from build123d import *

# Parameters (mm, degrees)
F0_W     = 370
F0_H     = 130
F1_DEPTH = 150
F2_T     = -10
F3_R     = 3
F4_DEPTH = 25


with BuildPart() as f1:
    # F0 (on Top) → F1 (new body)
    with BuildSketch(Plane.XY):
        Rectangle(F0_W, F0_H)
    extrude(amount=F1_DEPTH)

    # F2
    f2_openings = [f1.faces().sort_by_distance(p)[0] for p in [
        (0, 0, 150),
    ]]
    offset(amount=F2_T, openings=f2_openings)

    # F3 (on face) → F4 (cut)
    with BuildSketch(Plane(origin=(-185, 0, 0), x_dir=(0, -1, 0), z_dir=(-1, 0, 0))):
        with Locations((-25, 135)):
            Circle(F3_R)
        with Locations((25, 135)):
            Circle(F3_R)
    extrude(amount=-F4_DEPTH, mode=Mode.SUBTRACT)


solid = f1.part
Work out the finished part from the listing and answer in its coordinate system (mm). A direction names the side the tool comes from. Round coordinates to 2 decimals unless told otherwise and drop trailing zeros. Write each loop counter-clockwise with the first axis right and the second up, starting at its lowest first coordinate (ties: lowest second). Pieces come first, ordered by that corner, then holes. Notation, with made-up numbers: (-7, 39) - (41, 39) arc R19 cw to (41, 47) - close; hole circle Ø4 at (37, 49). An arc over 180 degrees is marked (long way). Answer in a Markdown table with one row per item. Add a question column.
1. A cutting plane is placed at C-C, the plane y = 12. Determine the outline of the cut face in (x, z), and give its area (3 significant figures).
2. Given pin 1 (4 mm diameter, centred on x = 75, y = -11, fed in from +Z); pin 2 (5 mm diameter, centred on y = 25, z = 135, fed in from -X), each flat-ended and moving along its own axis, determine where each tip first touches the part or whether it passes through.
3. A cutting plane is placed at B-B, the plane z = 117. Determine the outline of the cut face in (x, y), and give its area (3 significant figures).
4. For faces 5 (the flat face through (185, -1, 74)), 6 (the flat face through (-2, -55, 79)), determine the directions among +Z, -Z, +X, -X, +Y, -Y from which every point of the face is accessible in a straight line to the end or side of a thin tool.
5. Find the intervals of material crossed by line 1 along Y through (x, z) = (-177.25, 135); line 2 along X through (y, z) = (27.5, 94.5); line 3 along Z through (x, y) = (-177, -25), in increasing order. Write a range as from..to.
6. The mould has two halves that part along Y. Classify faces 1 (the flat face through (-2, 55, 79)), 2 (the flat face through (-3, 65, 74)), 3 (the flat face through (175, -1, 79)), 4 (the flat face through (-185, -1, 74)): +Y half, -Y half, draft (parallel to the pull), parting line (faces both ways), or undercut.
7. A cutting plane is placed at A-A, the plane x = 89. Determine the outline of the cut face in (y, z).
Worked out:
| question | item | result |
|---|---|---|
| 1 | outline | (-185, 0) - (185, 0) - (185, 150) - (175, 150) - (175, 10) - (-175, 10) - (-175, 150) - (-185, 150) - close |
| 1 | area | 6,500 mm^2 |
| 2 | pin 1 | z = 10 |
| 2 | pin 2 | x = 175 |
| 3 | outline | (-185, -65) - (185, -65) - (185, 65) - (-185, 65) - close; hole (-175, -55) - (175, -55) - (175, 55) - (-175, 55) - close |
| 3 | area | 9,600 mm^2 |
| 4 | face 5 | +Z, -Z, +X, +Y, -Y |
| 4 | face 6 | +Z |
| 5 | line 1 | -65..-28, -22..22, 28..65 |
| 5 | line 2 | -185..-175, 175..185 |
| 5 | line 3 | 0..132, 138..150 |
| 6 | face 1 | undercut |
| 6 | face 2 | +Y half |
| 6 | face 3 | undercut |
| 6 | face 4 | draft |
| 7 | outline | (-65, 0) - (65, 0) - (65, 150) - (55, 150) - (55, 10) - (-55, 10) - (-55, 150) - (-65, 150) - close |
